Read the model definition and answer for the solid it produces. Units are mm, in the model's axes. Face numbers are marked on the shaded views. A direction names the side the tool comes from. Coordinates: 2 decimals unless noted, no trailing zeros. Order: outer loops, then holes, each group sorted by start corner. A loop starts at its lowest first (then second) coordinate and runs counter-clockwise, first axis right, second up. Notation, with made-up numbers: (50, -36) -> (55, -36) arc R20 ccw to (55, -24) -> close; hole circle Ø3 at (75.5, -27). An arc over 180 degrees is marked (long way). Answer in a Markdown table with one row per item.
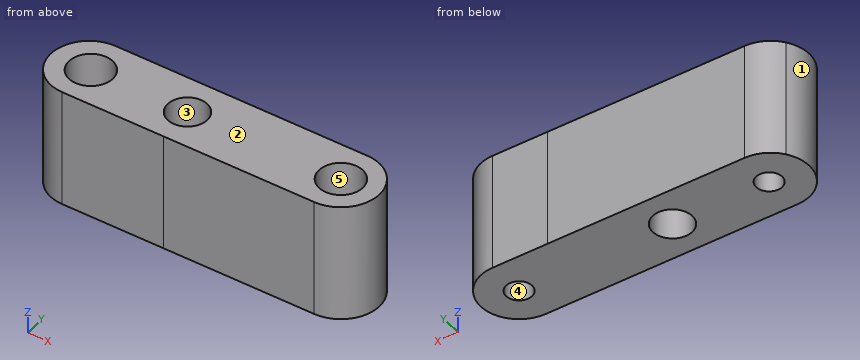
Solid Edge part; units mm, degrees
sketch "Sketch1" plane through (0, 0, 0) normal (0, 0, 1) x (1, 0, 0)
  circle A0 centre (-20.7647, 19.9) radius 2.2
  circle A1 centre (22.4644, 19.9) radius 2.2
  arc A2 (-26.3732, 23.6514) -> (-26.3732, 16.1486) centre (-20.9429, 19.9) ccw
  arc A3 (-26.3732, 16.1486) -> (-21.1336, 13.4) centre (-21.1336, 19.7683) ccw
  line L0 (-21.1336, 13.4) -> (-3.5966, 13.4)
  line L1 (-3.5966, 13.4) -> (2.9921, 13.4)
  line L2 (2.9921, 13.4) -> (22.4644, 13.4)
  arc A4 (22.4644, 13.4) -> (22.4644, 26.4) centre (22.4644, 19.9) ccw
  line L3 (22.4644, 26.4) -> (12.906, 26.4)
  line L4 (12.906, 26.4) -> (-21.1336, 26.4)
  arc A5 (-26.3732, 23.6514) -> (-21.1336, 26.4) centre (-21.1336, 20.0317) cw
extrude "Protrusion1" add sketch "Sketch1" along normal blind 20
sketch "Sketch2" plane through (0.7107, 19.9, 20) normal (0, 0, 1) x (1, 0, 0)
  circle A0 centre (-4.7754, 0.0168) radius 3.35
extrude "ExtrudedCutout_1" cut sketch "Sketch2" against normal blind 67.0154
sketch "Sketch3" plane through (0.7107, 19.9, 20) normal (0, 0, 1) x (1, 0, 0)
  circle A0 centre (-21.4754, 0) radius 3.7
  circle A1 centre (21.7537, 0) radius 3.7
extrude "ExtrudedCutout_2" cut sketch "Sketch3" against normal blind 14
Q1. The part is cut by section C-C (y = 14.5). Write down the section's boundary in (x, z).
Outcome:
| item | result |
|---|---|
| outline | (-24.71, 0) -> (26.08, 0) -> (26.08, 20) -> (-24.71, 20) -> close |
Q2. Given pin 1 (4 mm diameter, centred on y = 23, z = 8, fed in from +X); pin 2 (1.5 mm diameter, centred on y = 25, z = 13.5, fed in from -X); pin 3 (5.5 mm diameter, centred on x = -4.06, y = 19.92, fed in from -Z); pin 4 (5 mm diameter, centred on x = 22.46, y = 19.9, fed in from +Z), each flat-ended and moving along its own axis, determine where each tip first touches the part or whether it passes through.
Outcome:
| item | result |
|---|---|
| pin 1 | x = 28.87 |
| pin 2 | x = -25.9 |
| pin 3 | through |
| pin 4 | z = 6 |
Q3. For a pull along Y with two mould halves and no side action, classify the marked faces 1, 2 and 3 as pulls with the +Y half, pulls with the -Y half, needs draft (parallel to the pull), parting line crosses it, or undercut.
Outcome:
| item | result |
|---|---|
| face 1 | parting line crosses it |
| face 2 | needs draft |
| face 3 | undercut |
Q4. For the marked faces 4 and 5, determine the directions among +Z, -Z, +X, -X, +Y, -Y from which every point of the face is accessible in a straight line to the end or side of a thin tool.
Outcome:
| item | result |
|---|---|
| face 4 | +Z, -Z |
| face 5 | +Z |
Q5. The part is cut by section B-B (z = 7). Write down the section's boundary in (x, y), then the cut area to 3 significant figures.
Outcome:
| item | result |
|---|---|
| outline | (-26.37, 16.15) arc R6.37 ccw to (-21.13, 13.4) -> (-3.6, 13.4) -> (22.46, 13.4) arc R6.5 ccw to (22.46, 26.4) -> (12.91, 26.4) -> (-21.13, 26.4) arc R6.37 ccw to (-26.37, 23.65) arc R6.6 ccw to start; hole circle Ø7.4 at (-20.76, 19.9); hole circle Ø6.7 at (-4.06, 19.92); hole circle Ø7.4 at (22.46, 19.9) |
| area | 577 mm² |
Q6. Consider line 1 (X direction, y = 19.9, z = 1.4); line 2 (X direction, y = 17.5, z = 6.5); line 3 (Z direction, x = -21, y = 16.5). Determine where each line is inside the solid, lowest interval first.
Outcome:
| item | result |
|---|---|
| line 1 | -27.54 to -22.96, -18.56 to -7.41, -0.71 to 20.26, 24.66 to 28.96 |
| line 2 | -27.09 to -23.58, -17.95 to -6.38, -1.74 to 19.65, 25.28 to 28.51 |
| line 3 | 0 to 6 |
Q7. The part is cut by section A-A (y = 18.5). Write down the section's boundary in (x, z).
Outcome:
| item | result |
|---|---|
| outline | (-27.39, 0) -> (-22.46, 0) -> (-22.46, 6) -> (-24.19, 6) -> (-24.19, 20) -> (-27.39, 20) -> close; (-19.07, 0) -> (-7.1, 0) -> (-7.1, 20) -> (-17.34, 20) -> (-17.34, 6) -> (-19.07, 6) -> close; (-1.03, 0) -> (20.77, 0) -> (20.77, 6) -> (19.04, 6) -> (19.04, 20) -> (-1.03, 20) -> close; (24.16, 0) -> (28.81, 0) -> (28.81, 20) -> (25.89, 20) -> (25.89, 6) -> (24.16, 6) -> close |
